Verification items for this drawing (mm, ordinates from the low corner). A direction names the side the tool comes from. Coordinates: 2 decimals unless noted, no trailing zeros. Order: outer loops, then holes, each group sorted by start corner. A loop starts at its lowest first (then second) coordinate and runs counter-clockwise, first axis right, second up. Notation, with made-up numbers: (14.25, -11) -> (54.25, -11) arc R29 cw to (54.25, 19) -> close; hole circle Ø1 at (-23.5, 7.25). An arc over 180 degrees is marked (long way). Answer as CSV lines item,"result". Start each with the question number.
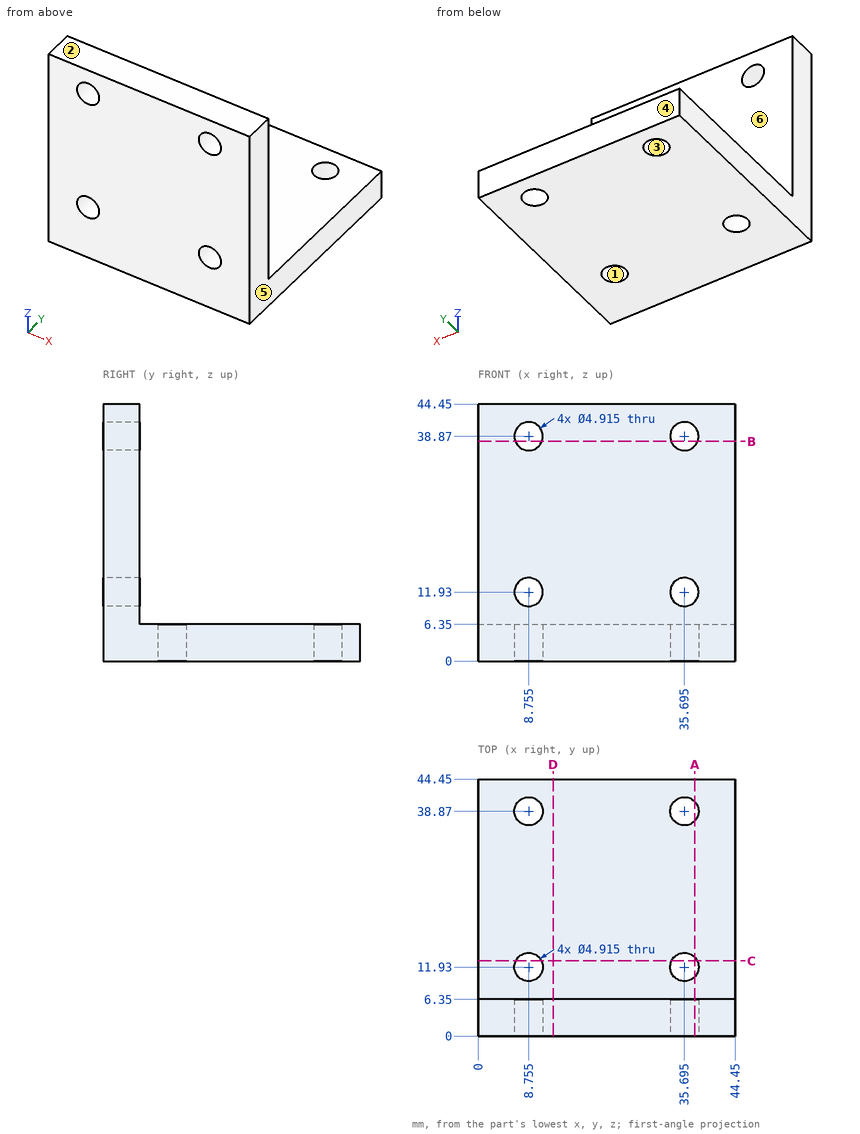
Q1. Sectioned sample at C-C, the plane y = 13. Record the cut outline in (x, z), then the cut area to 3 significant figures.
Q2. Sectioned sample at D-D, the plane x = 13. Record the cut outline in (y, z).
Q3. Release check for a two-part mould opening along Y. For the marked faces 1, 2, 3 and 4 record: released by +Y, released by -Y, zero draft, split by the parting line, or undercut.
Q4. Access from +Z, -Z, +X, -X, +Y, -Y to the whole of each face (thin tool, end or side, straight path). Record for the marked faces 5 and 6.
Q5. Thickness scan on L1, parallel to Y at x = 14, z = 28; L2, parallel to Y at x = 34.5, z = 3. Record the ranges inside material, lowest first.
Q6. Sectioned sample at A-A, the plane x = 37.5. Record the cut outline in (y, z).
Q7. Go/stop test with flat-tipped pins: pin 1 Ø6 at (x, y) = (39.5, 13.5) entering from +Z; pin 2 Ø11.5 at (x, z) = (23, 32.5) entering from +Y. Record where each tip stops, or that it passes through.
Q8. Sectioned sample at B-B, the plane z = 38. Record the cut outline in (x, y).
Geometry results:
1,outline,"(0, 0) -> (6.54, 0) -> (6.54, 6.35) -> (0, 6.35) -> close; (10.97, 0) -> (33.48, 0) -> (33.48, 6.35) -> (10.97, 6.35) -> close; (37.91, 0) -> (44.45, 0) -> (44.45, 6.35) -> (37.91, 6.35) -> close"
1,area,"226 mm^2"
2,outline,"(0, 0) -> (44.45, 0) -> (44.45, 6.35) -> (6.35, 6.35) -> (6.35, 44.45) -> (0, 44.45) -> close"
3,face 1,"undercut"
3,face 2,"zero draft"
3,face 3,"undercut"
3,face 4,"released by +Y"
4,face 5,"+Z, -Z, +X, +Y, -Y"
4,face 6,"+Z, +X, -X, +Y"
5,L1,"y = 0 to 6.35"
5,L2,"y = 0 to 9.78, 14.08 to 36.72, 41.02 to 44.45"
6,outline,"(0, 0) -> (10.26, 0) -> (10.26, 6.35) -> (6.35, 6.35) -> (6.35, 10.26) -> (0, 10.26) -> close; (0, 13.6) -> (6.35, 13.6) -> (6.35, 37.2) -> (0, 37.2) -> close; (0, 40.54) -> (6.35, 40.54) -> (6.35, 44.45) -> (0, 44.45) -> close; (13.6, 0) -> (37.2, 0) -> (37.2, 6.35) -> (13.6, 6.35) -> close; (40.54, 0) -> (44.45, 0) -> (44.45, 6.35) -> (40.54, 6.35) -> close"
7,pin 1,"stops at z = 6.35"
7,pin 2,"stops at y = 6.35"
8,outline,"(0, 0) -> (6.46, 0) -> (6.46, 6.35) -> (0, 6.35) -> close; (11.05, 0) -> (33.4, 0) -> (33.4, 6.35) -> (11.05, 6.35) -> close; (37.99, 0) -> (44.45, 0) -> (44.45, 6.35) -> (37.99, 6.35) -> close"
